```python
from build123d import *

# Parameters (mm, degrees)
ESQUISSE1_W                  = 70
ESQUISSE1_H                  = 70
BOSS_EXTRU_1_DEPTH           = 64
ESQUISSE2_W                  = 30.4
ESQUISSE2_H                  = 19.8
ESQUISSE2_H_2                = 30.4
ESQUISSE2_W_2                = 19.8
ENL_V_MAT_EXTRU_1_DEPTH      = 50
ESQUISSE5_W                  = 3
ESQUISSE5_H                  = 2
ENL_V_MAT_EXTRU_3_DEPTH      = 71
ESQUISSE6_W                  = 2
ESQUISSE6_H                  = 3
ENL_V_MAT_EXTRU_4_DEPTH      = 71
ESQUISSE7_R                  = 1
ENL_V_MAT_EXTRU_5_DEPTH      = 65
ENL_V_MAT_EXTRU_7_DEPTH      = 10
BOSS_EXTRU_2_DEPTH           = 3.8
ESQUISSE10_W                 = 27
ESQUISSE10_H                 = 18.1
ENL_V_MAT_EXTRU_8_DEPTH      = 10
ESQUISSE11_R                 = 1.25
ENL_V_MAT_EXTRU_9_DEPTH      = 15
R_P_TITION_CIRCULAIRE1_COUNT = 2


with BuildPart() as part:
    # Esquisse1 → Boss.-Extru.1 (new body)
    with BuildSketch(Plane.XY):
        with Locations((-35, 35)):
            Rectangle(ESQUISSE1_W, ESQUISSE1_H)
    extrude(amount=BOSS_EXTRU_1_DEPTH)

    # Esquisse2 → Enlèv. mat.-Extru.1 (cut)
    with BuildSketch(Plane.XY.offset(64)):
        with Locations((-35, 60.1)):
            Rectangle(ESQUISSE2_W, ESQUISSE2_H)
        with Locations((-35, 35)):
            Rectangle(ESQUISSE2_W, ESQUISSE2_H_2)
        with Locations((-9.9, 35)):
            Rectangle(ESQUISSE2_W_2, ESQUISSE2_H_2)
        with Locations((-60.1, 35)):
            Rectangle(ESQUISSE2_W_2, ESQUISSE2_H_2)
        with Locations((-35, 9.9)):
            Rectangle(ESQUISSE2_W, ESQUISSE2_H)
    extrude(amount=-ENL_V_MAT_EXTRU_1_DEPTH, mode=Mode.SUBTRACT)

    # Esquisse5 → Enlèv. mat.-Extru.3 (cut, through all)
    with BuildSketch(Plane.ZY.offset(70)):
        with Locations((59.5, 69)):
            Rectangle(ESQUISSE5_W, ESQUISSE5_H)
        with Locations((59.5, 1)):
            Rectangle(ESQUISSE5_W, ESQUISSE5_H)
    extrude(amount=-ENL_V_MAT_EXTRU_3_DEPTH, mode=Mode.SUBTRACT)

    # Esquisse6 → Enlèv. mat.-Extru.4 (cut, through all)
    with BuildSketch(Plane(origin=(0, 70, 0), x_dir=(1, 0, 0), z_dir=(0, 1, 0))):
        with Locations((-69, -59.5)):
            Rectangle(ESQUISSE6_W, ESQUISSE6_H)
    extrude(amount=-ENL_V_MAT_EXTRU_4_DEPTH, mode=Mode.SUBTRACT)

    # Esquisse7 → Enlèv. mat.-Extru.5 (cut, through all)
    with BuildSketch(Plane.XY.offset(64)):
        with Locations((-52.2, 17.8)):
            Circle(ESQUISSE7_R)
    enl_v_mat_extru_5 = extrude(amount=-ENL_V_MAT_EXTRU_5_DEPTH, mode=Mode.SUBTRACT)

    # Esquisse8 → Enlèv. mat.-Extru.7 (cut)
    with BuildSketch(Plane(origin=(0, 0, 0), x_dir=(-1, 0, 0), z_dir=(0, 0, -1))):
        with BuildLine():
            Line((60.2, 0), (60.2, 17.8))
            ThreePointArc((60.2, 17.8), (52.2, 9.8), (44.2, 17.8))
            Line((44.2, 17.8), (44.2, 0))
            Line((44.2, 0), (60.2, 0))
        make_face()
        with BuildLine():
            ThreePointArc((44.2, 17.8), (52.2, 9.8), (60.2, 17.8))
            Line((60.2, 17.8), (53.2, 17.8))
            ThreePointArc((53.2, 17.8), (52.2, 16.8), (51.2, 17.8))
            Line((51.2, 17.8), (44.2, 17.8))
        make_face()
        with BuildLine():
            Line((53.2, 17.8), (60.2, 17.8))
            ThreePointArc((60.2, 17.8), (52.2, 25.8), (44.2, 17.8))
            Line((44.2, 17.8), (51.2, 17.8))
            ThreePointArc((51.2, 17.8), (52.2, 18.8), (53.2, 17.8))
        make_face()
    enl_v_mat_extru_7 = extrude(amount=-ENL_V_MAT_EXTRU_7_DEPTH, mode=Mode.SUBTRACT)

    # Esquisse9 → Boss.-Extru.2 (add)
    with BuildSketch(Plane(origin=(0, 0, 0), x_dir=(-1, 0, 0), z_dir=(0, 0, -1))):
        with BuildLine():
            Line((46.2, 0), (46.2, 17.8))
            ThreePointArc((46.2, 17.8), (52.2, 23.8), (58.2, 17.8))
            Line((58.2, 17.8), (58.2, 0))
            Line((58.2, 0), (60.2, 0))
            Line((60.2, 0), (60.2, 17.8))
            Line((60.2, 17.8), (60.175717696, 28.742363645))
            Line((60.175717696, 28.742363645), (44.2, 28.742363645))
            Line((44.2, 28.742363645), (44.2, 0))
            Line((44.2, 0), (46.2, 0))
        make_face()
    extrude(amount=-BOSS_EXTRU_2_DEPTH)

    # Esquisse10 → Enlèv. mat.-Extru.8 (cut)
    with BuildSketch(Plane(origin=(0, 0, 0), x_dir=(-1, 0, 0), z_dir=(0, 0, -1))):
        with Locations((52.2, 9.05)):
            Rectangle(ESQUISSE10_W, ESQUISSE10_H)
    enl_v_mat_extru_8 = extrude(amount=-ENL_V_MAT_EXTRU_8_DEPTH, mode=Mode.SUBTRACT)

    # Esquisse11 → Enlèv. mat.-Extru.9 (cut)
    with BuildSketch(Plane.XZ.offset(-18.1)):
        with Locations(Location((-41.7, 7, 0), (0, 0, 270))):  # turned: the seam where the file's is
            Circle(ESQUISSE11_R)
        with Locations(Location((-62.7, 7, 0), (0, 0, 270))):  # turned: the seam where the file's is
            Circle(ESQUISSE11_R)
    extrude(amount=-ENL_V_MAT_EXTRU_9_DEPTH, mode=Mode.SUBTRACT)

    # Répétition circulaire1: Enlèv. mat.-Extru.5, Enlèv. mat.-Extru.7, Enlèv. mat.-Extru.8 ×2 about axis
    r_p_tition_circulaire1_axis = Axis((-35, 35, 0), (0, 0, 1))
    add([enl_v_mat_extru_5.rotate(r_p_tition_circulaire1_axis, i * 360 / R_P_TITION_CIRCULAIRE1_COUNT) for i in range(1, R_P_TITION_CIRCULAIRE1_COUNT)], mode=Mode.SUBTRACT)
    add([enl_v_mat_extru_7.rotate(r_p_tition_circulaire1_axis, i * 360 / R_P_TITION_CIRCULAIRE1_COUNT) for i in range(1, R_P_TITION_CIRCULAIRE1_COUNT)], mode=Mode.SUBTRACT)
    add([enl_v_mat_extru_8.rotate(r_p_tition_circulaire1_axis, i * 360 / R_P_TITION_CIRCULAIRE1_COUNT) for i in range(1, R_P_TITION_CIRCULAIRE1_COUNT)], mode=Mode.SUBTRACT)


solid = part.part
```
CAD build for the part. Positions are in the model's coordinates, mm. A direction names the side the tool comes from. Coordinates: 2 decimals unless noted, no trailing zeros. Order: outer loops, then holes, each group sorted by start corner. A loop starts at its lowest first (then second) coordinate and runs counter-clockwise, first axis right, second up.
(1) Saw through at B-B, the plane x = -17.8. Write the cut outline in (y, z).
Solution:
outline: (0, 0) - (44.2, 0) - (44.2, 10) - (51.2, 10) - (51.2, 64) - (50.2, 64) - (50.2, 14) - (19.8, 14) - (19.8, 64) - (0, 64) - (0, 61) - (2, 61) - (2, 58) - (0, 58) - close; (53.2, 10) - (70, 10) - (70, 58) - (68, 58) - (68, 61) - (70, 61) - (70, 64) - (53.2, 64) - close
(2) Saw through at D-D, the plane x = -41.7. Write the cut outline in (y, z).
Solution:
outline: (0, 10) - (18.1, 10) - (18.1, 8.25) - (33.1, 8.25) - (33.1, 5.75) - (18.1, 5.75) - (18.1, 0) - (70, 0) - (70, 14) - (0, 14) - close
(3) Saw through at A-A, the plane z = 48.5. Write the cut outline in (x, y), and give its area (3 significant figures).
Solution:
outline: (-70, 0) - (-50.2, 0) - (-50.2, 19.8) - (-70, 19.8) - close; (-70, 50.2) - (-50.2, 50.2) - (-50.2, 70) - (-70, 70) - close; (-19.8, 0) - (0, 0) - (0, 19.8) - (-19.8, 19.8) - close; (-19.8, 50.2) - (0, 50.2) - (0, 70) - (-19.8, 70) - close; hole circle Ø2 at (-52.2, 17.8); hole circle Ø2 at (-17.8, 52.2)
area: 1,560 mm2
(4) Saw through at C-C, the plane y = 57.5. Write the cut outline in (x, z), and give its area (3 significant figures).
Solution:
outline: (-70, 0) - (-31.3, 0) - (-31.3, 10) - (-4.3, 10) - (-4.3, 0) - (0, 0) - (0, 64) - (-19.8, 64) - (-19.8, 14) - (-50.2, 14) - (-50.2, 64) - (-70, 64) - (-70, 61) - (-68, 61) - (-68, 58) - (-70, 58) - close
area: 2,680 mm2
(5) Which spindle directions (+Z, -Z, +X, -X, +Y, -Y) get a long thin tool onto all of the face, cutting with end or side? Do faces 4 (the face through (-10, 68, 59)), 5 (the face through (-50.2, 10, 39)), 6 (the face through (-68, 11, 60)). Say none if no direction does.
Solution:
face 4: +X, -X, +Y
face 5: +Z, +Y, -Y
face 6: -X, +Y, -Y
(6) Pin check, flat tips, straight feed: pin 1 Ø10 at (y, z) = (10.5, 44.5) entering from +X; pin 2 Ø4 at (x, y) = (-49, 22) entering from +Z; pin 3 Ø3 at (x, z) = (-63.5, 7.5) entering from -Y. Stop position of each tip, or through.
Solution:
pin 1: stops at x = 0
pin 2: stops at z = 14
pin 3: stops at y = 18.1
(7) Drill centre lines: L1, parallel to Y at x = -52.2, z = 39; L2, parallel to X at y = 52.2, z = 23; L3, parallel to X at y = 27, z = 7. Where is each one in solid material? Low to high.
Solution:
L1: y = 0 to 16.8, 18.8 to 19.8, 50.2 to 70
L2: x = -70 to -50.2, -19.8 to -18.8, -16.8 to 0
L3: x = -70 to -63.95, -61.45 to -42.95, -40.45 to 0
(8) Mould opens along X. For faces 1 (the face through (-70, 60, 62)), 2 (the face through (-63.92, 25.5, 7.27)), 3 (the face through (-68.2, 63.7, 58)) say: released by +X, released by -X, zero draft, split by the parting line, or undercut.
Solution:
face 1: released by -X
face 2: undercut
face 3: zero draft
